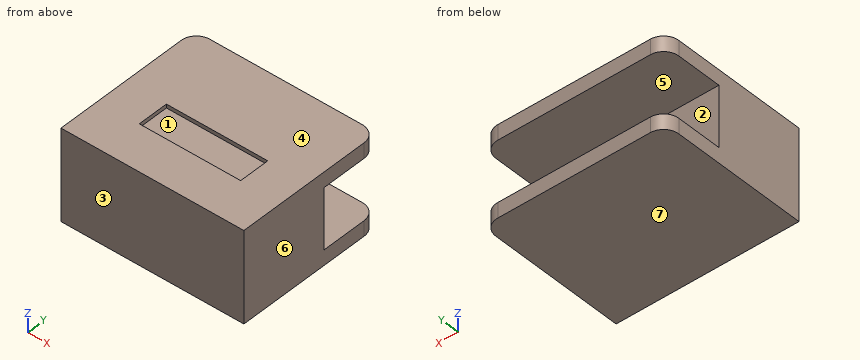
from build123d import *

# Parameters (mm, degrees)
SKETCH1_W           = 152.4
SKETCH1_H           = 76.2
BOSS_EXTRUDE1_DEPTH = 76.2
SKETCH2_W           = 152.4
SKETCH2_H           = 12.7
BOSS_EXTRUDE2_DEPTH = 50.8
FILLET1_R           = 12.7
SKETCH3_W           = 84.462045133
SKETCH3_H           = 25.769420555
CUT_EXTRUDE1_DEPTH  = 3.175


with BuildPart() as part:
    # Sketch1 → Boss-Extrude1 (new body)
    with BuildSketch(Plane.XY):
        with Locations((76.2, 38.1)):
            Rectangle(SKETCH1_W, SKETCH1_H)
    extrude(amount=BOSS_EXTRUDE1_DEPTH)

    # Sketch2 → Boss-Extrude2 (add)
    with BuildSketch(Plane(origin=(0, 76.2, 0), x_dir=(1, 0, 0), z_dir=(0, 1, 0))):
        with Locations((76.2, -6.35)):
            Rectangle(SKETCH2_W, SKETCH2_H)
    boss_extrude2 = extrude(amount=BOSS_EXTRUDE2_DEPTH)

    # Mirror1: Boss-Extrude2 across plane
    add(boss_extrude2.mirror(Plane.XY.offset(38.1)))

    # Fillet1
    fillet1_edges = [part.edges().sort_by_distance(p)[0] for p in [
        (0, 127, 6.35),
        (152.4, 127, 6.35),
        (0, 127, 69.85),
        (152.4, 127, 69.85),
    ]]
    fillet(fillet1_edges, radius=FILLET1_R)

    # Sketch3 → Cut-Extrude1 (cut)
    with BuildSketch(Plane.XY.offset(76.2)):
        with Locations((76.416893198, 48.36205359)):
            Rectangle(SKETCH3_W, SKETCH3_H)
    extrude(amount=-CUT_EXTRUDE1_DEPTH, mode=Mode.SUBTRACT)


solid = part.part
Build history of the part. All positions in model axes, mm. Face numbers are marked on the shaded views. A direction names the side the tool comes from. Coordinates: 2 decimals unless noted, no trailing zeros. Write each loop counter-clockwise with the first axis right and the second up, starting at its lowest first coordinate (ties: lowest second). Pieces come first, ordered by that corner, then holes. Notation, with made-up numbers: (56.25, 2) -> (109.25, 2) arc R25 cw to (109.25, 23) -> close; hole circle Ø8 at (-31, 40). An arc over 180 degrees is marked (long way). Use CSV: the item, a comma, the result in double quotes. Start each with the question number.
Q1. Cut at C-C, the plane y = 54. List the corners of the cut face in (x, z) (3 decimals).
Q2. 3-axis set-ups, long thin cutter, end or side, ignore diameter. For the marked faces 1, 2 and 3: which of +Z, -Z, +X, -X, +Y, -Y reach the whole face in a straight line?
Q3. Cut at D-D, the plane z = 15.5. List the corners of the cut face in (x, y), then the cut area to 3 significant figures.
Q4. Drill centre lines: probe 1 along Z at (x, y) = (57, 79); probe 2 along Y at (x, z) = (91.5, 47.5); probe 3 along Z at (x, y) = (96, 54.5) (3 decimals). Where is each one in solid material? Low to high.
Q5. Pull direction Z, two halves, no side cores. Call the marked faces 4, 5, 6 and 7: released by +Z, released by -Z, zero draft, split by the parting line, or undercut.
Q6. Cut at B-B, the plane x = 25. List the corners of the cut face in (y, z).
Q7. Flat gauge pin, fed straight in: pin 1 Ø2 at (x, z) = (104.5, 48.5) entering from +Y. Where does the tip first touch, or does it go through?
Q8. Cut at A-A, the plane y = 100. List the corners of the cut face in (x, z), then the cut area to 3 significant figures.
Checked values:
1,outline,"(0, 0) -> (152.4, 0) -> (152.4, 76.2) -> (118.648, 76.2) -> (118.648, 73.025) -> (34.186, 73.025) -> (34.186, 76.2) -> (0, 76.2) -> close"
2,face 1,"+Z"
2,face 2,"+X, -X, +Y"
2,face 3,"+Z, -Z, +X, -X, -Y"
3,outline,"(0, 0) -> (152.4, 0) -> (152.4, 76.2) -> (0, 76.2) -> close"
3,area,"11,600 mm²"
4,probe 1,"z = 0 to 12.7, 63.5 to 76.2"
4,probe 2,"y = 0 to 76.2"
4,probe 3,"z = 0 to 73.025"
5,face 4,"released by +Z"
5,face 5,"undercut"
5,face 6,"zero draft"
5,face 7,"released by -Z"
6,outline,"(0, 0) -> (127, 0) -> (127, 12.7) -> (76.2, 12.7) -> (76.2, 63.5) -> (127, 63.5) -> (127, 76.2) -> (0, 76.2) -> close"
7,pin 1,"stops at y = 76.2"
8,outline,"(0, 0) -> (152.4, 0) -> (152.4, 12.7) -> (0, 12.7) -> close; (0, 63.5) -> (152.4, 63.5) -> (152.4, 76.2) -> (0, 76.2) -> close"
8,area,"3,870 mm²"
